Answer from the drawing. Dimensions are ordinates in mm from the lowest x, y and z of the part. A direction names the side the tool comes from. Round coordinates to 2 decimals unless told otherwise and drop trailing zeros. Loops run counter-clockwise (first coordinate to the right, second up) from the corner with the lowest first, then second, coordinate; pieces in that order, holes last. Notation, with made-up numbers: (-8, -22) - (7, -22) arc R13 cw to (7, 3) - close; hole circle Ø4 at (4.25, -10.75). An arc over 180 degrees is marked (long way). Return JSON: item names as keys, results as strings.
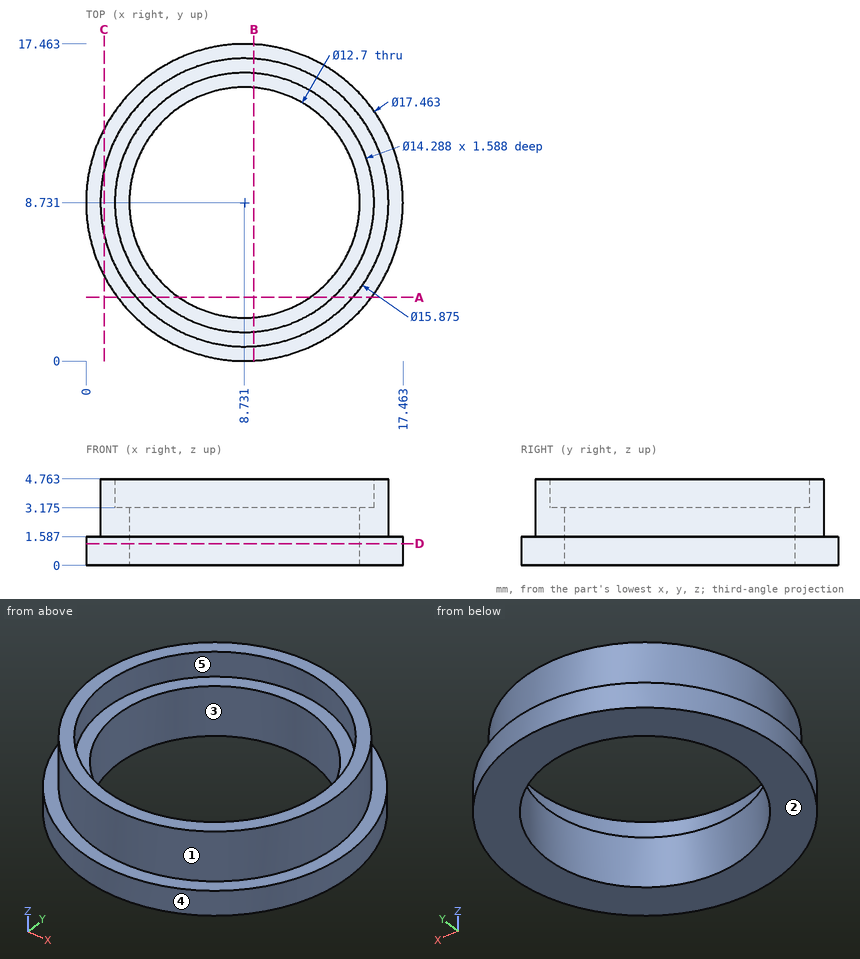
1) Flat-ended cylindrical pins translate along their axes: pin 1 (8 mm diameter, centred on x = 10.5, y = 11.5, fed in from -Z); pin 2 (1.5 mm diameter, centred on x = 4, z = 3.5, fed in from +Y); pin 3 (3 mm diameter, centred on x = 4.5, y = 10, fed in from +Z). Find the tip coordinate at first contact, or state that the pin passes through.
Verdict:
{"pin 1": "stops at z = 0", "pin 2": "stops at y = 15.6", "pin 3": "passes through"}
2) Determine the mould class of the marked faces 1, 2 and 3 for opening direction Y: pulls with the +Y half, pulls with the -Y half, needs draft (parallel to the pull), parting line crosses it, or undercut.
Verdict:
{"face 1": "parting line crosses it", "face 2": "needs draft", "face 3": "undercut"}
3) Section C-C (x = 1) is taken. Give the vertices of the cut face in (y, z), and give its area (3 significant figures).
Verdict:
{"outline": "(4.67, 0) - (12.79, 0) - (12.79, 1.59) - (10.53, 1.59) - (10.53, 4.76) - (6.93, 4.76) - (6.93, 1.59) - (4.67, 1.59) - close", "area": "24.3 mm2"}
4) Section A-A (y = 3.5) is taken. Give the vertices of the cut face in (x, z) (1 decimal).
Verdict:
{"outline": "(1.7, 0) - (5.1, 0) - (5.1, 3.2) - (3.9, 3.2) - (3.9, 4.8) - (2.8, 4.8) - (2.8, 1.6) - (1.7, 1.6) - close; (12.3, 0) - (15.7, 0) - (15.7, 1.6) - (14.7, 1.6) - (14.7, 4.8) - (13.6, 4.8) - (13.6, 3.2) - (12.3, 3.2) - close"}
5) Section B-B (x = 9.25) is taken. Give the vertices of the cut face in (y, z) (1 decimal).
Verdict:
{"outline": "(0, 0) - (2.4, 0) - (2.4, 3.2) - (1.6, 3.2) - (1.6, 4.8) - (0.8, 4.8) - (0.8, 1.6) - (0, 1.6) - close; (15.1, 0) - (17.4, 0) - (17.4, 1.6) - (16.7, 1.6) - (16.7, 4.8) - (15.9, 4.8) - (15.9, 3.2) - (15.1, 3.2) - close"}
6) Section D-D (z = 1.2) is taken. Give the vertices of the cut face in (x, y), and give its area (3 significant figures).
Verdict:
{"outline": "circle Ø17.46 at (8.73, 8.73); hole circle Ø12.7 at (8.73, 8.73)", "area": "113 mm2"}
7) A tool of negligible diameter and unlimited length cuts with its end or side. For the marked faces 4 and 5, from which of +Z, -Z, +X, -X, +Y, -Y can it reach the whole face along a straight path? Write none if from no direction.
Verdict:
{"face 4": "+Z, -Z", "face 5": "+Z"}
8) Find the intervals of material crossed by L1, parallel to X at y = 8.5, z = 1.55 (1 decimal); L2, parallel to Z at x = 13.25, y = 13.25 (1 decimal), in increasing order.
Verdict:
{"L1": "x = 0 to 2.4, 15.1 to 17.5", "L2": "z = 0 to 3.2"}
